Part model, mm, in its own coordinate system. Face numbers are marked on the shaded views. A direction names the side the tool comes from. Give positions to 0.01 mm unless a question says otherwise; leave off trailing zeros. Loops run counter-clockwise (first coordinate to the right, second up) from the corner with the lowest first, then second, coordinate; pieces in that order, holes last. Notation, with made-up numbers: (79.5, 87) -> (111.5, 87) arc R23 cw to (111.5, 117) -> close; hole circle Ø10 at (-39, 85.25). An arc over 180 degrees is marked (long way). One line per question, with ' | ' between items.
```python
from build123d import *

# Parameters (mm, degrees)
Y_KSEKLIK_EKSTR_ZYON2_DEPTH = 10
RADYUS1_R                   = 0.8


with BuildPart() as part:
    # Çizim3 → Yükseklik-Ekstrüzyon2 (new body)
    with BuildSketch(Plane.XY):
        with BuildLine():
            Line((1, 0), (6.1, 0))
            Line((6.1, 0), (6.1, 0.5))
            Line((6.1, 0.5), (6.85, 0.5))
            Line((6.85, 0.5), (6.85, 1.4))
            Line((6.85, 1.4), (4.321320344, 1.4))
            ThreePointArc((4.321320344, 1.4), (3.582216718, 1.893853254), (3.755634919, 2.765685425))
            Line((3.755634919, 2.765685425), (7.638403375, 6.648453882))
            ThreePointArc((7.638403375, 6.648453882), (10, 5.9), (12.361596625, 6.648453882))
            Line((12.361596625, 6.648453882), (16.244365081, 2.765685425))
            ThreePointArc((16.244365081, 2.765685425), (16.417783282, 1.893853254), (15.678679656, 1.4))
            Line((15.678679656, 1.4), (13.15, 1.4))
            Line((13.15, 1.4), (13.15, 0.5))
            Line((13.15, 0.5), (13.9, 0.5))
            Line((13.9, 0.5), (13.9, 0))
            Line((13.9, 0), (26.1, 0))
            Line((26.1, 0), (26.1, 0.5))
            Line((26.1, 0.5), (26.85, 0.5))
            Line((26.85, 0.5), (26.85, 1.4))
            Line((26.85, 1.4), (24.321320344, 1.4))
            ThreePointArc((24.321320344, 1.4), (23.582216718, 1.893853254), (23.755634919, 2.765685425))
            Line((23.755634919, 2.765685425), (27.638403375, 6.648453882))
            ThreePointArc((27.638403375, 6.648453882), (30, 5.9), (32.361596625, 6.648453882))
            Line((32.361596625, 6.648453882), (36.244365081, 2.765685425))
            ThreePointArc((36.244365081, 2.765685425), (36.417783282, 1.893853254), (35.678679656, 1.4))
            Line((35.678679656, 1.4), (33.15, 1.4))
            Line((33.15, 1.4), (33.15, 0.5))
            Line((33.15, 0.5), (33.9, 0.5))
            Line((33.9, 0.5), (33.9, 0))
            Line((33.9, 0), (39, 0))
            ThreePointArc((39, 0), (39.707106781, 0.292893219), (40, 1))
            Line((40, 1), (40, 6.1))
            Line((40, 6.1), (39.5, 6.1))
            Line((39.5, 6.1), (39.5, 6.85))
            Line((39.5, 6.85), (38.6, 6.85))
            Line((38.6, 6.85), (38.6, 4.321320344))
            ThreePointArc((38.6, 4.321320344), (38.106146746, 3.582216718), (37.234314575, 3.755634919))
            Line((37.234314575, 3.755634919), (33.351546118, 7.638403375))
            ThreePointArc((33.351546118, 7.638403375), (34.1, 10), (33.351546118, 12.361596625))
            Line((33.351546118, 12.361596625), (37.234314575, 16.244365081))
            ThreePointArc((37.234314575, 16.244365081), (38.106146746, 16.417783282), (38.6, 15.678679656))
            Line((38.6, 15.678679656), (38.6, 13.15))
            Line((38.6, 13.15), (39.5, 13.15))
            Line((39.5, 13.15), (39.5, 13.9))
            Line((39.5, 13.9), (40, 13.9))
            Line((40, 13.9), (40, 19))
            ThreePointArc((40, 19), (39.707106781, 19.707106781), (39, 20))
            Line((39, 20), (33.9, 20))
            Line((33.9, 20), (33.9, 19.5))
            Line((33.9, 19.5), (33.15, 19.5))
            Line((33.15, 19.5), (33.15, 18.6))
            Line((33.15, 18.6), (35.678679656, 18.6))
            ThreePointArc((35.678679656, 18.6), (36.417783282, 18.106146746), (36.244365081, 17.234314575))
            Line((36.244365081, 17.234314575), (32.361596625, 13.351546118))
            ThreePointArc((32.361596625, 13.351546118), (30, 14.1), (27.638403375, 13.351546118))
            Line((27.638403375, 13.351546118), (23.755634919, 17.234314575))
            ThreePointArc((23.755634919, 17.234314575), (23.582216718, 18.106146746), (24.321320344, 18.6))
            Line((24.321320344, 18.6), (26.85, 18.6))
            Line((26.85, 18.6), (26.85, 19.5))
            Line((26.85, 19.5), (26.1, 19.5))
            Line((26.1, 19.5), (26.1, 20))
            Line((26.1, 20), (13.9, 20))
            Line((13.9, 20), (13.9, 19.5))
            Line((13.9, 19.5), (13.15, 19.5))
            Line((13.15, 19.5), (13.15, 18.6))
            Line((13.15, 18.6), (15.678679656, 18.6))
            ThreePointArc((15.678679656, 18.6), (16.417783282, 18.106146746), (16.244365081, 17.234314575))
            Line((16.244365081, 17.234314575), (12.361596625, 13.351546118))
            ThreePointArc((12.361596625, 13.351546118), (10, 14.1), (7.638403375, 13.351546118))
            Line((7.638403375, 13.351546118), (3.755634919, 17.234314575))
            ThreePointArc((3.755634919, 17.234314575), (3.582216718, 18.106146746), (4.321320344, 18.6))
            Line((4.321320344, 18.6), (6.85, 18.6))
            Line((6.85, 18.6), (6.85, 19.5))
            Line((6.85, 19.5), (6.1, 19.5))
            Line((6.1, 19.5), (6.1, 20))
            Line((6.1, 20), (1, 20))
            ThreePointArc((1, 20), (0.292893219, 19.707106781), (0, 19))
            Line((0, 19), (0, 13.9))
            Line((0, 13.9), (0.5, 13.9))
            Line((0.5, 13.9), (0.5, 13.15))
            Line((0.5, 13.15), (1.4, 13.15))
            Line((1.4, 13.15), (1.4, 15.678679656))
            ThreePointArc((1.4, 15.678679656), (1.893853254, 16.417783282), (2.765685425, 16.244365081))
            Line((2.765685425, 16.244365081), (6.648453882, 12.361596625))
            ThreePointArc((6.648453882, 12.361596625), (5.9, 10), (6.648453882, 7.638403375))
            Line((6.648453882, 7.638403375), (2.765685425, 3.755634919))
            ThreePointArc((2.765685425, 3.755634919), (1.893853254, 3.582216718), (1.4, 4.321320344))
            Line((1.4, 4.321320344), (1.4, 6.85))
            Line((1.4, 6.85), (0.5, 6.85))
            Line((0.5, 6.85), (0.5, 6.1))
            Line((0.5, 6.1), (0, 6.1))
            Line((0, 6.1), (0, 1))
            ThreePointArc((0, 1), (0.292893219, 0.292893219), (1, 0))
        make_face()
        with BuildLine():
            Line((21.210320913, 18.6), (18.789679087, 18.6))
            ThreePointArc((18.789679087, 18.6), (18.223993662, 18.365685425), (17.989679087, 17.8))
            Line((17.989679087, 17.8), (17.989679087, 17.331100443))
            ThreePointArc((17.989679087, 17.331100443), (17.928782713, 17.024953697), (17.755364512, 16.765415018))
            Line((17.755364512, 16.765415018), (13.351546118, 12.361596625))
            ThreePointArc((13.351546118, 12.361596625), (14.1, 10), (13.351546118, 7.638403375))
            Line((13.351546118, 7.638403375), (17.755364512, 3.234584982))
            ThreePointArc((17.755364512, 3.234584982), (17.928782713, 2.975046303), (17.989679087, 2.668899557))
            Line((17.989679087, 2.668899557), (17.989679087, 2.2))
            ThreePointArc((17.989679087, 2.2), (18.223993662, 1.634314575), (18.789679087, 1.4))
            Line((18.789679087, 1.4), (21.210320913, 1.4))
            ThreePointArc((21.210320913, 1.4), (21.776006338, 1.634314575), (22.010320913, 2.2))
            Line((22.010320913, 2.2), (22.010320913, 2.668899557))
            ThreePointArc((22.010320913, 2.668899557), (22.071217287, 2.975046303), (22.244635488, 3.234584982))
            Line((22.244635488, 3.234584982), (26.648453882, 7.638403375))
            ThreePointArc((26.648453882, 7.638403375), (25.9, 10), (26.648453882, 12.361596625))
            Line((26.648453882, 12.361596625), (22.244635488, 16.765415018))
            ThreePointArc((22.244635488, 16.765415018), (22.071217287, 17.024953697), (22.010320913, 17.331100443))
            Line((22.010320913, 17.331100443), (22.010320913, 17.8))
            ThreePointArc((22.010320913, 17.8), (21.776006338, 18.365685425), (21.210320913, 18.6))
        make_face(mode=Mode.SUBTRACT)
        with BuildLine():
            Line((8.201142588, 12.443783276), (8.552743846, 12.092182018))
            ThreePointArc((8.552743846, 12.092182018), (10, 12.543968548), (11.447256154, 12.092182018))
            Line((11.447256154, 12.092182018), (11.798857412, 12.443783276))
            ThreePointArc((11.798857412, 12.443783276), (12.443783276, 12.443783276), (12.443783276, 11.798857412))
            Line((12.443783276, 11.798857412), (12.092182018, 11.447256154))
            ThreePointArc((12.092182018, 11.447256154), (12.543968548, 10), (12.092182018, 8.552743846))
            Line((12.092182018, 8.552743846), (12.443783276, 8.201142588))
            ThreePointArc((12.443783276, 8.201142588), (12.443783276, 7.556216724), (11.798857412, 7.556216724))
            Line((11.798857412, 7.556216724), (11.447256154, 7.907817982))
            ThreePointArc((11.447256154, 7.907817982), (10, 7.456031452), (8.552743846, 7.907817982))
            Line((8.552743846, 7.907817982), (8.201142588, 7.556216724))
            ThreePointArc((8.201142588, 7.556216724), (7.556216724, 7.556216724), (7.556216724, 8.201142588))
            Line((7.556216724, 8.201142588), (7.907817982, 8.552743846))
            ThreePointArc((7.907817982, 8.552743846), (7.456031452, 10), (7.907817982, 11.447256154))
            Line((7.907817982, 11.447256154), (7.556216724, 11.798857412))
            ThreePointArc((7.556216724, 11.798857412), (7.556216724, 12.443783276), (8.201142588, 12.443783276))
        make_face(mode=Mode.SUBTRACT)
        with BuildLine():
            Line((27.907817982, 11.447256154), (27.556216724, 11.798857412))
            ThreePointArc((27.556216724, 11.798857412), (27.556216724, 12.443783276), (28.201142588, 12.443783276))
            Line((28.201142588, 12.443783276), (28.552743846, 12.092182018))
            ThreePointArc((28.552743846, 12.092182018), (30, 12.543968548), (31.447256154, 12.092182018))
            Line((31.447256154, 12.092182018), (31.798857412, 12.443783276))
            ThreePointArc((31.798857412, 12.443783276), (32.443783276, 12.443783276), (32.443783276, 11.798857412))
            Line((32.443783276, 11.798857412), (32.092182018, 11.447256154))
            ThreePointArc((32.092182018, 11.447256154), (32.543968548, 10), (32.092182018, 8.552743846))
            Line((32.092182018, 8.552743846), (32.443783276, 8.201142588))
            ThreePointArc((32.443783276, 8.201142588), (32.443783276, 7.556216724), (31.798857412, 7.556216724))
            Line((31.798857412, 7.556216724), (31.447256154, 7.907817982))
            ThreePointArc((31.447256154, 7.907817982), (30, 7.456031452), (28.552743846, 7.907817982))
            Line((28.552743846, 7.907817982), (28.201142588, 7.556216724))
            ThreePointArc((28.201142588, 7.556216724), (27.556216724, 7.556216724), (27.556216724, 8.201142588))
            Line((27.556216724, 8.201142588), (27.907817982, 8.552743846))
            ThreePointArc((27.907817982, 8.552743846), (27.456031452, 10), (27.907817982, 11.447256154))
        make_face(mode=Mode.SUBTRACT)
    extrude(amount=Y_KSEKLIK_EKSTR_ZYON2_DEPTH)

    # Radyus1
    radyus1_edges = [part.edges().sort_by_distance(p)[0] for p in [
        (6.648453882, 7.638403375, 5),
        (6.648453882, 12.361596625, 5),
        (33.351546118, 12.361596625, 5),
        (33.351546118, 7.638403375, 5),
        (13.351546118, 12.361596625, 5),
        (13.351546118, 7.638403375, 5),
        (26.648453882, 7.638403375, 5),
        (26.648453882, 12.361596625, 5),
    ]]
    fillet(radyus1_edges, radius=RADYUS1_R)


solid = part.part
```
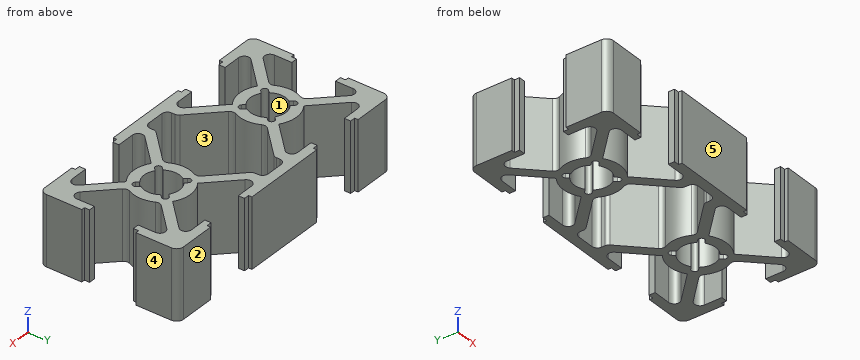
1) Saw through at A-A (y = 9.5). Give the cut face in (x, z).
Found:
outline: (5.93, 0) -> (7.51, 0) -> (7.51, 10) -> (5.93, 10) -> close; (12.49, 0) -> (14.07, 0) -> (14.07, 10) -> (12.49, 10) -> close; (25.93, 0) -> (27.51, 0) -> (27.51, 10) -> (25.93, 10) -> close; (32.49, 0) -> (34.07, 0) -> (34.07, 10) -> (32.49, 10) -> close
2) Pin check, flat tip, straight feed: P1, Ø1, axis at y = 9.5, z = 5.5, coming from the -X side. Stop position of the tip, or through.
Found:
P1: x = 5.9
3) Tool access for the marked faces 1 and 2: list every direction of +Z, -Z, +X, -X, +Y, -Y with a clear straight run to the whole face (end or side of a thin tool).
Found:
face 1: +Z, -Z | face 2: +Z, -Z, +X, -X, +Y
4) Saw through at B-B (y = 15.25). Give the cut face in (x, z).
Found:
outline: (0, 0) -> (1.4, 0) -> (1.4, 10) -> (0, 10) -> close; (3.76, 0) -> (5.74, 0) -> (5.74, 10) -> (3.76, 10) -> close; (14.26, 0) -> (16.24, 0) -> (16.24, 10) -> (14.26, 10) -> close; (23.76, 0) -> (25.74, 0) -> (25.74, 10) -> (23.76, 10) -> close; (34.26, 0) -> (36.24, 0) -> (36.24, 10) -> (34.26, 10) -> close; (38.6, 0) -> (40, 0) -> (40, 10) -> (38.6, 10) -> close
5) Drill centre lines: line 1 (Y direction, x = 20, z = 3); line 2 (Y direction, x = 25, z = 3.5); line 3 (Y direction, x = 15.5, z = 7). Where is each one in solid material? Low to high.
Found:
line 1: 0 to 1.4, 18.6 to 20 | line 2: 0 to 1.4, 4.01 to 5.99, 14.01 to 15.99, 18.6 to 20 | line 3: 0 to 1.4, 3.51 to 5.49, 14.51 to 16.49, 18.6 to 20
6) Saw through at C-C (z = 1). State how many separate pieces and enclosed holes the cut face has, and give its area (3 significant figures).
Found:
separate pieces: 1 | enclosed holes: 3 | area: 255 mm2
7) Pull direction X, two halves, no side cores. Call the marked faces 3, 4 and 5: pulls with the +X half, pulls with the -X half, needs draft (parallel to the pull), parting line crosses it, or undercut.
Found:
face 3: undercut | face 4: pulls with the +X half | face 5: needs draft
